The drawing under review shows one solid part. Ordinate dimensions are in mm from its lowest x, y, z. Coordinates: 2 decimals unless noted, no trailing zeros. Order: outer loops, then holes, each group sorted by start corner. A loop starts at its lowest first (then second) coordinate and runs counter-clockwise, first axis right, second up.
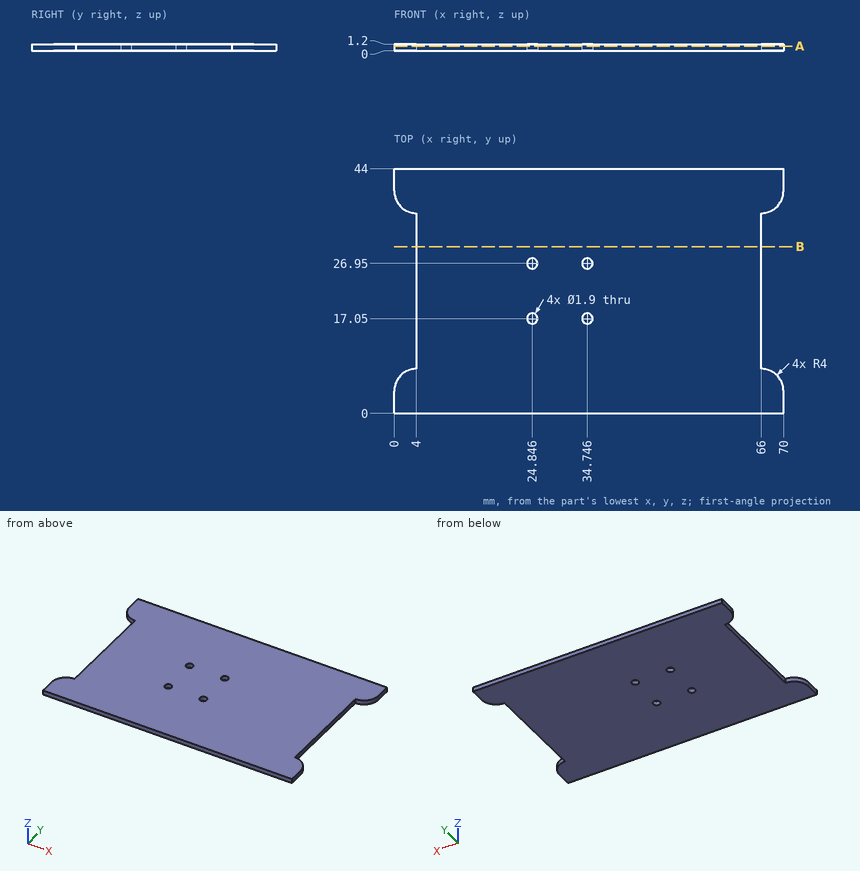
1. To check wall thickness, follow L1, parallel to X at y = 17, z = 0.2 (1 decimal); L2, parallel to X at y = 19, z = 0.45; L3, parallel to X at y = 7.5, z = 0.7 (1 decimal). State the ranges of each line that lie inside material, in increasing order.
Answer below:
L1: x = 4 to 23.9, 25.8 to 33.8, 35.7 to 66
L2: x = 4 to 66
L3: x = 2.1 to 67.9
2. Take a section at A-A, the plane z = 0.8. Give the number of separate pieces and of enclosed holes in the cut face, plus the area to 3 significant figures.
Answer below:
separate pieces: 1
enclosed holes: 4
area: 2,830 mm2
3. Take a section at B-B, the plane y = 30. Give the boundary of the cut face in (x, z).
Answer below:
outline: (4, 0) - (66, 0) - (66, 1.2) - (4, 1.2) - close
